Read the model definition and answer for the solid it produces. Units are mm, in the model's axes. Coordinates: 2 decimals unless noted, no trailing zeros. Write each loop counter-clockwise with the first axis right and the second up, starting at its lowest first coordinate (ties: lowest second). Pieces come first, ordered by that corner, then holes. Notation, with made-up numbers: (80.5, 80) -> (85.5, 80) arc R16 cw to (85.5, 91) -> close; hole circle Ø2 at (65, -16). An arc over 180 degrees is marked (long way). One line per item, written item: value. Start each with the question number.
1. Find section A-A, the plane z = 4.15. Write down the section's boundary in (x, y) (1 decimal), and give its area (3 significant figures).
2. Given P1, Ø5, axis at x = -8, y = -0.5, coming from the +Z side, flat-ended and moving along its own axis, determine where the tip first touches the part or whether it passes through.
3. Consider line 1 along Y through (x, z) = (13.5, 4.7) (3 decimals); line 2 along X through (y, z) = (2, 4.2); line 3 along Z through (x, y) = (10, -0.75). Determine where each line is inside the solid, lowest interval first.
4. Find section C-C, the plane y = 1. Write down the section's boundary in (x, z), and give its area (3 significant figures).
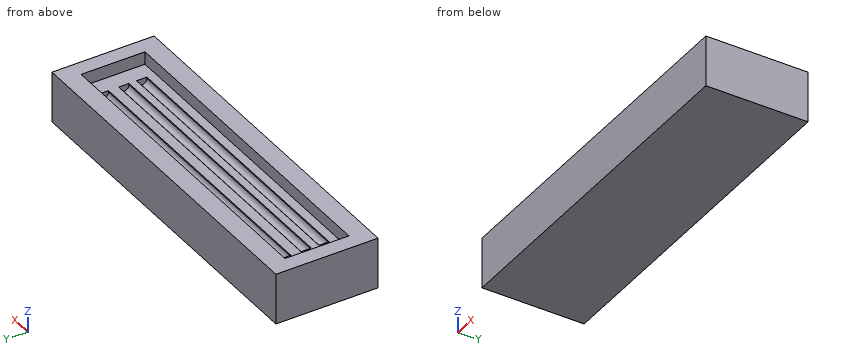
```python
from build123d import *

# Parameters (mm, degrees)
F0_W     = 35.56
F0_H     = 10.16
F1_DEPTH = 5.08
F2_W     = 32.385
F2_H     = 6.35
F3_DEPTH = 1.27
F4_W     = 28.956
F4_H     = 1.016
F5_DEPTH = 0.635
F6_R     = 0.50799


# Not quite as in the source:
# - a fillet or chamfer is up to 0.001 mm smaller than in the source, because OpenCascade refuses the exact size


with BuildPart() as f1:
    # F0 (on Top) → F1 (new body)
    with BuildSketch(Plane.XY):
        Rectangle(F0_W, F0_H)
    extrude(amount=F1_DEPTH)

    # F2 (on face) → F3 (cut)
    with BuildSketch(Plane.XY.offset(5.08)):
        Rectangle(F2_W, F2_H)
    extrude(amount=-F3_DEPTH, mode=Mode.SUBTRACT)

    # F4 (on face) → F5 (cut)
    with BuildSketch(Plane.XY.offset(3.81)):
        Rectangle(F4_W, F4_H)
        with Locations((0, 2.032)):
            Rectangle(F4_W, F4_H)
        with Locations((0, -1.778)):
            Rectangle(F4_W, F4_H)
    extrude(amount=-F5_DEPTH, mode=Mode.SUBTRACT)

    # F6 (radius 0.508 in the source; OpenCascade refuses exactly that, so slightly less here)
    f6_edges = [f1.edges().sort_by_distance(p)[0] for p in [
        (0, 0.508, 3.175),
        (0, -0.508, 3.175),
        (0, 2.54, 3.175),
        (0, -1.27, 3.175),
        (0, 1.524, 3.175),
        (0, -2.286, 3.175),
    ]]
    fillet(f6_edges, radius=F6_R)


solid = f1.part
```
Answer block:
1. outline: (-17.8, -5.1) -> (17.8, -5.1) -> (17.8, 5.1) -> (-17.8, 5.1) -> close; hole (-16.2, -3.2) -> (16.2, -3.2) -> (16.2, 3.2) -> (-16.2, 3.2) -> close
1. area: 156 mm2
2. P1: stops at z = 3.81
3. line 1: y = -5.08 to -3.175, 3.175 to 5.08
3. line 2: x = -17.78 to -16.19, 16.19 to 17.78
3. line 3: z = 0 to 3.81
4. outline: (-17.78, 0) -> (17.78, 0) -> (17.78, 5.08) -> (16.19, 5.08) -> (16.19, 3.81) -> (-16.19, 3.81) -> (-16.19, 5.08) -> (-17.78, 5.08) -> close
4. area: 140 mm2
